The listing builds one solid part. Answer for the finished solid, in the listing's coordinates (mm). Coordinates: 2 decimals unless noted, no trailing zeros. Write each loop counter-clockwise with the first axis right and the second up, starting at its lowest first coordinate (ties: lowest second). Pieces come first, ordered by that corner, then holes. Notation, with made-up numbers: M 52.25,60.25 L 73.25,60.25 A25 ccw 73.25,84.25 Z; hole C 85,34 d5. An arc over 180 degrees is marked long. Write item = value, one per line. Start each with the question number.
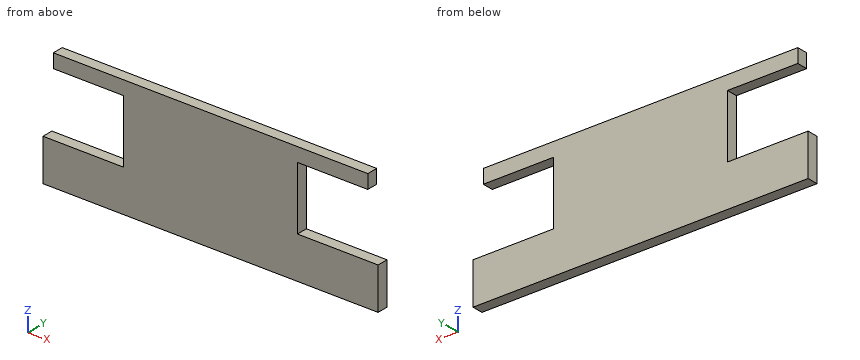
```python
from build123d import *

# Parameters (mm, degrees)
SKETCH1_W         = 48.84
SKETCH1_H         = 17.34
MAIN_SQUARE_DEPTH = 1.6
SKETCH2_W         = 1.5
SKETCH2_H         = 2.04
SERVO_HOLES_DEPTH = 1.6


with BuildPart() as part:
    # Sketch1 → main square (new body)
    with BuildSketch(Plane(origin=(0, 0, 0), x_dir=(1, 0, 0), z_dir=(0, 1, 0))):
        with Locations((24.42, 8.67)):
            Rectangle(SKETCH1_W, SKETCH1_H)
    extrude(amount=MAIN_SQUARE_DEPTH)

    # Sketch2 → servo holes (cut)
    with BuildSketch(Plane(origin=(0, 1.6, 0), x_dir=(1, 0, 0), z_dir=(0, 1, 0))):
        Polygon((11.75, 11.24), (0, 11.24), (0, 2.04), (1.5, 2.04), (11.75, 2.04), align=None)
        with Locations((0.75, 1.02)):
            Rectangle(SKETCH2_W, SKETCH2_H)
    servo_holes = extrude(amount=-SERVO_HOLES_DEPTH, mode=Mode.SUBTRACT)

    # Mirror1: servo holes across plane
    add(servo_holes.mirror(Plane.ZY.offset(-24.42)), mode=Mode.SUBTRACT)


solid = part.part
```
1. The part is cut by section A-A, the plane x = 10.5. Write down the section's boundary in (y, z).
2. Straight lines are drawn through the part: L1, parallel to Z at x = 9, y = 1.35; L2, parallel to X at y = 0.85, z = -5.75; L3, parallel to X at y = 1.25, z = -1.5. For each, find the intervals that lie inside material, in ascending order. Write a range as [from, to].
3. The part is cut by section C-C, the plane z = -10.25. Write down the section's boundary in (x, y).
4. Each of these flat-tipped pins is pushed along its axis until it touches: pin 1 (2 mm diameter, centred on x = 43.5, z = -9, fed in from -Y); pin 2 (10 mm diameter, centred on x = 18, z = -7, fed in from -Y); pin 3 (0.5 mm diameter, centred on y = 1, z = -1, fed in from -X). Where does it stop, or does it pass through?
5. The part is cut by section B-B, the plane y = 1.05. Write down the section's boundary in (x, z), and give its area (3 significant figures).
Solution:
q1.outline = M 0,-17.34 L 1.6,-17.34 L 1.6,-11.24 L 0,-11.24 Z; M 0,-2.04 L 1.6,-2.04 L 1.6,0 L 0,0 Z
q2.L1 = [-17.34, -11.24], [-2.04, 0]
q2.L2 = [11.75, 37.09]
q2.L3 = [1.5, 47.34]
q3.outline = M 11.75,0 L 37.09,0 L 37.09,1.6 L 11.75,1.6 Z
q4.pin_1 = through
q4.pin_2 = 0
q4.pin_3 = 1.5
q5.outline = M 0,-17.34 L 48.84,-17.34 L 48.84,-11.24 L 37.09,-11.24 L 37.09,-2.04 L 47.34,-2.04 L 47.34,0 L 1.5,0 L 1.5,-2.04 L 11.75,-2.04 L 11.75,-11.24 L 0,-11.24 Z
q5.area = 625 mm^2
